from build123d import *

# Parameters (mm, degrees)
SKETCH1_R           = 6.35
BOSS_EXTRUDE1_DEPTH = 6.35
SKETCH2_R           = 6.35
BOSS_EXTRUDE3_DEPTH = 25.4
SKETCH5_R           = 2.54
CUT_EXTRUDE2_DEPTH  = 118.774954893


with BuildPart() as part:
    # Sketch1 → Boss-Extrude1 (new body)
    with BuildSketch(Plane.XY):
        with BuildLine():
            Line((-12.7, -101.6), (-12.7, 101.6))
            ThreePointArc((-12.7, 101.6), (0, 114.3), (12.7, 101.6))
            Line((12.7, 101.6), (12.7, -101.6))
            ThreePointArc((12.7, -101.6), (0, -114.3), (-12.7, -101.6))
        make_face()
        with Locations((0, 101.6)):
            Circle(SKETCH1_R, mode=Mode.SUBTRACT)
        with Locations(Location((0, -101.6, 0), (0, 0, 180))):
            Circle(SKETCH1_R, mode=Mode.SUBTRACT)
    extrude(amount=BOSS_EXTRUDE1_DEPTH)

    # Sketch2 → Boss-Extrude3 (add)
    with BuildSketch(Plane.XY):
        with Locations((0, 101.6)):
            Circle(SKETCH2_R)
    extrude(amount=BOSS_EXTRUDE3_DEPTH)

    # Sketch5 → Cut-Extrude2 (cut, through all)
    with BuildSketch(Plane(origin=(0, 0, 0), x_dir=(1, 0, 0), z_dir=(0, 1, 0))):
        with Locations(Location((0, -15.875, 0), (0, 0, 90))):
            Circle(SKETCH5_R)
    extrude(amount=CUT_EXTRUDE2_DEPTH, mode=Mode.SUBTRACT)


solid = part.part
Could you check a few things on this model? Use its own coordinates, in mm. A direction names the side the tool comes from. Give positions to 0.01 mm unless a question says otherwise; leave off trailing zeros. Order: outer loops, then holes, each group sorted by start corner. A loop starts at its lowest first (then second) coordinate and runs counter-clockwise, first axis right, second up.
1. Suppose I cut it at B-B (z = 2.75). Write out the boundary of the cut face in (x, y).
Answers below:
outline: (-12.7, -101.6) arc R12.7 ccw to (12.7, -101.6) - (12.7, 101.6) arc R12.7 ccw to (-12.7, 101.6) - close; hole circle Ø12.7 at (0, -101.6)
2. For pin 1 (10 mm diameter, centred on x = -0.5, z = 9, fed in from +Y); pin 2 (5 mm diameter, centred on x = -10, y = 80, fed in from +Z); pin 3 (8 mm diameter, centred on x = -2, z = 13.5, fed in from -Y), each with a flat end and sliding along its axis, tell me the tip position at first contact or that it passes through.
Answers below:
pin 1: stops at y = 114.3
pin 2: stops at z = 6.35
pin 3: stops at y = 95.25
3. Suppose I cut it at A-A (x = 0). Write out the boundary of the cut face in (y, z) (3 decimals), plus the area to 3 significant figures.
Answers below:
outline: (-114.3, 0) - (-107.95, 0) - (-107.95, 6.35) - (-114.3, 6.35) - close; (-95.25, 0) - (114.3, 0) - (114.3, 6.35) - (107.95, 6.35) - (107.95, 13.335) - (95.25, 13.335) - (95.25, 6.35) - (-95.25, 6.35) - close; (95.25, 18.415) - (107.95, 18.415) - (107.95, 25.4) - (95.25, 25.4) - close
area: 1,550 mm2
4. Suppose I cut it at C-C (y = 53). Write out the boundary of the cut face in (x, z).
Answers below:
outline: (-12.7, 0) - (12.7, 0) - (12.7, 6.35) - (-12.7, 6.35) - close
5. I need wall thicknesses on L1, parallel to X at y = -101.6, z = 2; L2, parallel to Y at x = 0, z = 4.25; L3, parallel to Z at x = -0.5, y = 33.5. Which ranges of each line are inside material? Lowest first, please.
Answers below:
L1: x = -12.7 to -6.35, 6.35 to 12.7
L2: y = -114.3 to -107.95, -95.25 to 114.3
L3: z = 0 to 6.35
6. Which directions (+Z, -Z, +X, -X, +Y, -Y) give clear straight access to the entire face, cutting with the end or side of a thin tool? Please do faces 5 (the cylindrical face through (2.93, 95.966, 15.742)), 6 (the flat face through (12.7, 1, 3)).
Answers below:
face 5: +Z
face 6: +Z, -Z, +X, +Y, -Y
7. Thinking about a two-plate mould opening in Y: for faces 1 (the cylindrical face through (0.8, -107.9, 3.1)), 2 (the flat face through (0, 2, 6.35)), 3 (the cylindrical face through (0.279, -114.297, 3.131)), 4 (the cylindrical face through (-0.279, 114.297, 3.131)), which applies, +Y half, -Y half, draft (parallel to the pull), parting line (faces both ways), or undercut?
Answers below:
face 1: undercut
face 2: draft
face 3: -Y half
face 4: +Y half
